```python
from build123d import *

# Parameters (mm, degrees)
SKETCH1_W           = 29.64084851
SKETCH1_H           = 22.995210284
BOSS_EXTRUDE1_DEPTH = 11
SKETCH2_W           = 11
SKETCH2_H           = 25.30011898
BOSS_EXTRUDE2_DEPTH = 10
CHAMFER1_SIZE       = 2
SKETCH3_W           = 31.444464136
SKETCH3_H           = 13.690550156
CUT_EXTRUDE2_DEPTH  = 6
SKETCH4_W           = 16.801230495
SKETCH4_H           = 6.210132239
BOSS_EXTRUDE3_DEPTH = 10
SKETCH5_R           = 2.040999549
CUT_EXTRUDE3_DEPTH  = 22.016469246
SKETCH6_W           = 4.621469737
SKETCH6_H           = 13.3986797
CUT_EXTRUDE4_DEPTH  = 16
SKETCH7_R           = 1.7
CUT_EXTRUDE5_DEPTH  = 27
SKETCH21_W          = 6.4100694
SKETCH21_H          = 8.3354859
BOSS_EXTRUDE4_DEPTH = 11
SKETCH20_W          = 6.410069378
SKETCH20_H          = 8.335485858
BOSS_EXTRUDE5_DEPTH = 11
CUT_EXTRUDE6_DEPTH  = 2.5
SKETCH19_R          = 1.7
CUT_EXTRUDE7_DEPTH  = 16
CUT_EXTRUDE8_DEPTH  = 2.5
SKETCH18_R          = 1.7
CUT_EXTRUDE9_DEPTH  = 16


with BuildPart() as part:
    # Sketch1 → Boss-Extrude1 (new body)
    with BuildSketch(Plane(origin=(0, 0, 0), x_dir=(0, 0, -1), z_dir=(1, 0, 0))):
        Rectangle(SKETCH1_W, SKETCH1_H)
    extrude(amount=BOSS_EXTRUDE1_DEPTH)

    # Sketch2 → Boss-Extrude2 (add)
    with BuildSketch(Plane(origin=(0, 11.497605142, 0), x_dir=(1, 0, 0), z_dir=(0, 1, 0))):
        with Locations((5.5, -2.170364765)):
            Rectangle(SKETCH2_W, SKETCH2_H)
    extrude(amount=BOSS_EXTRUDE2_DEPTH)

    # Chamfer1
    chamfer1_edges = [part.edges().sort_by_distance(p)[0] for p in [
        (5.5, 21.497605142, -10.479694725),
        (5.5, 21.497605142, 14.820424255),
        (5.5, 11.497605142, -14.820424255),
    ]]
    chamfer(chamfer1_edges, length=CHAMFER1_SIZE)

    # Sketch3 → Cut-Extrude2 (cut)
    with BuildSketch(Plane.ZY):
        with Locations((0.26445091, 0.38357275)):
            Rectangle(SKETCH3_W, SKETCH3_H)
    extrude(amount=-CUT_EXTRUDE2_DEPTH, mode=Mode.SUBTRACT)

    # Sketch4 → Boss-Extrude3 (add)
    with BuildSketch(Plane(origin=(6, 0.435062227, 0), x_dir=(0, 0, 1), z_dir=(-1, 0, 0))):
        with Locations((-2.204570257, -0.002306757)):
            Rectangle(SKETCH4_W, SKETCH4_H)
    extrude(amount=BOSS_EXTRUDE3_DEPTH)

    # Sketch5 → Cut-Extrude3 (cut, through all)
    with BuildSketch(Plane.XY.offset(6.196044991)):
        with Locations((0.212787141, 0.369675098)):
            Circle(SKETCH5_R)
    extrude(amount=-CUT_EXTRUDE3_DEPTH, mode=Mode.SUBTRACT)

    # Sketch6 → Cut-Extrude4 (cut, through all)
    with BuildSketch(Plane(origin=(11, 0, 0), x_dir=(0, 0, -1), z_dir=(1, 0, 0))):
        with Locations((2.429578273, 0.383063563)):
            Rectangle(SKETCH6_W, SKETCH6_H)
    extrude(amount=-CUT_EXTRUDE4_DEPTH, mode=Mode.SUBTRACT)

    # Sketch7 → Cut-Extrude5 (cut)
    with BuildSketch(Plane.XY.offset(14.820424255)):
        with Locations((5.312142967, 15.762432364)):
            Circle(SKETCH7_R)
    extrude(amount=-CUT_EXTRUDE5_DEPTH, mode=Mode.SUBTRACT)

    # Sketch21 → Boss-Extrude4 (add)
    with BuildSketch(Plane(origin=(11, 0, 0), x_dir=(0, 0, -1), z_dir=(1, 0, 0))):
        with Locations((10.097369078, -7.290376311)):
            Rectangle(SKETCH21_W, SKETCH21_H)
    extrude(amount=-BOSS_EXTRUDE4_DEPTH)

    # Sketch20 → Boss-Extrude5 (add)
    with BuildSketch(Plane(origin=(11, 0, 0), x_dir=(0, 0, -1), z_dir=(1, 0, 0))):
        with Locations((-10.015073396, -7.232029734)):
            Rectangle(SKETCH20_W, SKETCH20_H)
    extrude(amount=-BOSS_EXTRUDE5_DEPTH)

    # Sketch15 → Cut-Extrude6 (cut)
    with BuildSketch(Plane(origin=(11, 0, 0), x_dir=(0, 0, -1), z_dir=(1, 0, 0))):
        Polygon((-8.109817508, -10.532029734), (-6.204561619, -7.232029734), (-8.109817508, -3.932029734), (-11.920329284, -3.932029734), (-13.825585173, -7.232029734), (-11.920329284, -10.532029734), align=None)
    extrude(amount=-CUT_EXTRUDE6_DEPTH, mode=Mode.SUBTRACT)

    # Sketch19 → Cut-Extrude7 (cut, through all)
    with BuildSketch(Plane(origin=(11, 0, 0), x_dir=(0, 0, -1), z_dir=(1, 0, 0))):
        with Locations((-10.015073396, -7.232029734)):
            Circle(SKETCH19_R)
    extrude(amount=-CUT_EXTRUDE7_DEPTH, mode=Mode.SUBTRACT)

    # Sketch17 → Cut-Extrude8 (cut)
    with BuildSketch(Plane(origin=(11, 0, 0), x_dir=(0, 0, -1), z_dir=(1, 0, 0))):
        Polygon((12.002624966, -10.590376311), (13.907880854, -7.290376311), (12.002624966, -3.990376311), (8.192113189, -3.990376311), (6.286857301, -7.290376311), (8.192113189, -10.590376311), align=None)
    extrude(amount=-CUT_EXTRUDE8_DEPTH, mode=Mode.SUBTRACT)

    # Sketch18 → Cut-Extrude9 (cut, through all)
    with BuildSketch(Plane(origin=(11, 0, 0), x_dir=(0, 0, -1), z_dir=(1, 0, 0))):
        with Locations((10.097369078, -7.290376311)):
            Circle(SKETCH18_R)
    extrude(amount=-CUT_EXTRUDE9_DEPTH, mode=Mode.SUBTRACT)


solid = part.part
```
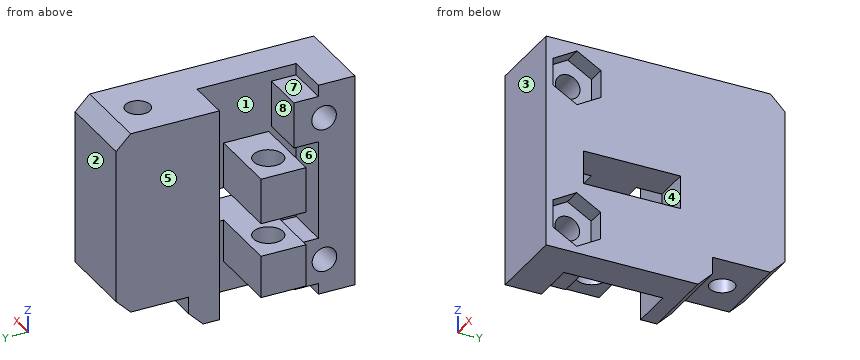
The model under review builds one solid part; all positions refer to its coordinate system, in mm. Face numbers are marked on the shaded views. A direction names the side the tool comes from. Round coordinates to 2 decimals unless told otherwise and drop trailing zeros. Write each loop counter-clockwise with the first axis right and the second up, starting at its lowest first coordinate (ties: lowest second). Pieces come first, ordered by that corner, then holes.
(1) Insertion check: pin 1 (1.2 mm diameter, centred on x = 6.5, z = -11, fed in from +Y); pin 2 (8 mm diameter, centred on y = 15.5, z = 4, fed in from -X); pin 3 (2.5 mm diameter, centred on x = 5.31, y = 15.76, fed in from -Z); pin 4 (2.5 mm diameter, centred on x = 2.5, y = -4.5, fed in from -Z). Each pin has a flat end and moves straight along its axis. Give the tip position at first contact, or say it passes through.
(2) We need section A-A on y = 4. Give the boundary of the cut face in (x, z).
(3) We need section D-D on z = -7.5. Give the boundary of the cut face in (x, y).
(4) Mouldability with a two-part tool opening along Y and no side actions: class the marked faces 1, 2 and 3 as +Y half, -Y half, draft (parallel to the pull), parting line (faces both ways), or undercut.
(5) Machinability: for the marked faces 4, 5, 6, 7 and 8, which of the approach directions +Z, -Z, +X, -X, +Y, -Y give a long, thin tool a straight path to every point of the face, cutting with its end or side? Answer none if there is none.
(6) We need section C-C on z = 9.25. Give the boundary of the cut face in (x, y), and give its area (3 significant figures).
(7) Wall thickness on L1, parallel to Y at x = 5.25, z = 0; L2, parallel to Y at x = 2.75, z = 6; L3, parallel to Z at x = 8, y = -4: over which ranges is each line inside the solid? List them lowest first.
(8) We need section B-B on x = -2.75. Give the boundary of the cut face in (y, z), and give its area (3 significant figures).
Findings below:
1. pin 1: stops at y = 19.58
1. pin 2: stops at x = 0
1. pin 3: passes through
1. pin 4: stops at z = -13.3
2. outline: (6, -14.82) - (11, -14.82) - (11, -4.74) - (6, -4.74) - close; (6, -0.12) - (11, -0.12) - (11, 14.82) - (6, 14.82) - close
3. outline: (-4, -2.67) - (6, -2.67) - (6, -3.12) - (0, -3.12) - (0, -11.5) - (11, -11.5) - (11, -9.39) - (8.5, -9.39) - (8.5, -5.19) - (11, -5.19) - (11, 21.5) - (0, 21.5) - (0, 7.23) - (6, 7.23) - (6, 3.54) - (-4, 3.54) - close; hole circle Ø4.08 at (0.21, 0.37); hole circle Ø3.4 at (5.31, 15.76)
4. face 1: undercut
4. face 2: +Y half
4. face 3: -Y half
5. face 4: +X, -X
5. face 5: +Z, -Z, -X, +Y
5. face 6: -X
5. face 7: +Z, -X
5. face 8: +Z, -Z, -X
6. outline: (0, -11.5) - (11, -11.5) - (11, -10.53) - (8.5, -10.53) - (8.5, -8.75) - (0, -8.75) - close; (0, -5.71) - (8.5, -5.71) - (8.5, -3.93) - (11, -3.93) - (11, 21.5) - (0, 21.5) - (0, 7.23) - (6, 7.23) - (6, -3.06) - (0, -3.06) - close; hole circle Ø3.4 at (5.31, 15.76)
6. area: 250 mm2
7. L1: y = -11.5 to -6.46, -2.67 to 3.54, 7.23 to 14.06, 17.46 to 21.5
7. L2: y = -11.5 to -6.46, -2.67 to 3.54, 7.23 to 21.5
7. L3: z = -14.82 to -4.74, -0.12 to 14.82
8. outline: (-2.67, -10.61) - (3.54, -10.61) - (3.54, -4.74) - (-2.67, -4.74) - close; (-2.67, -0.12) - (3.54, -0.12) - (3.54, 6.2) - (-2.67, 6.2) - close
8. area: 75.6 mm2
